The listing builds one solid part. Answer for the finished solid, in the listing's coordinates (mm). A direction names the side the tool comes from. Round coordinates to 2 decimals unless told otherwise and drop trailing zeros. Loops run counter-clockwise (first coordinate to the right, second up) from the corner with the lowest first, then second, coordinate; pieces in that order, holes last. Notation, with made-up numbers: M -31,82 L -12,82 A37 ccw -12,119 Z; hole C 82.25,-26.5 d4. An arc over 180 degrees is marked long. Put each result on its own line as item: value. Start each with the question number.
(1) Section D-D, the plane y = -30.5 is taken. Determine the outline of the cut face in (x, z), then the cut area to 3 significant figures.
(2) Flat-ended cylindrical pins translate along their axes: P1, Ø1.5, axis at y = 24, z = 3, coming from the +X side; P2, Ø1.5, axis at x = -12.5, z = 4, coming from the +Y side; P3, Ø2.5, axis at y = -23.5, z = 2.5, coming from the +X side. Find the tip coordinate at first contact, or state that the pin passes through.
(3) Section B-B, the plane y = -22 is taken. Determine the outline of the cut face in (x, z), then the cut area to 3 significant figures.
(4) Straight lines are drawn through the part: line 1 (Y direction, x = -0.5, z = 2.8) (3 decimals); line 2 (Y direction, x = 2, z = 4.75); line 3 (X direction, y = 12.5, z = 0.2) (3 decimals). For each, find the intervals that lie inside material, in ascending order.
(5) Determine the mould class of faces 3 (the face through (25, -2, 2)), 4 (the face through (0, 21.5, 3)), 5 (the face through (17.482, 29.871, 2.535)), 6 (the face through (-20.982, -28.273, 2.535)) for opening direction Y: released by +Y, released by -Y, zero draft, split by the parting line, or undercut.
(6) Section A-A, the plane z = 1.4 is taken. Count the separate pieces of the cut face and the enclosed holes in it, then the cut area to 3 significant figures.
(7) Section C-C, the plane x = -19.5 is taken. Determine the outline of the cut face in (y, z).
(8) Which of the six approach directions +Z, -Z, +X, -X, +Y, -Y give full straight-line access (tool end or side, diameter ignored) to faces 1 (the face through (-25, -2, 2)), 2 (the face through (3.5, -24, 3))?
```python
from build123d import *

# Parameters (mm, degrees)
SKETCH1_R           = 37
BOSS_EXTRUDE1_DEPTH = 5
CUT_EXTRUDE3_START  = -10
CUT_EXTRUDE3_DEPTH  = 10
FILLET2_R           = 25
FILLET3_R           = 20
SKETCH7_W           = 5
SKETCH7_H           = 5
SKETCH7_W_2         = 7
CUT_EXTRUDE4_DEPTH  = 10
SKETCH8_W           = 10
SKETCH8_H           = 7
CUT_EXTRUDE5_DEPTH  = 10


with BuildPart() as part:
    # Sketch1 → Boss-Extrude1 (new body)
    with BuildSketch(Plane.XY):
        Circle(SKETCH1_R)
    extrude(amount=BOSS_EXTRUDE1_DEPTH)

    # Sketch6 → Cut-Extrude3 (cut)
    with BuildSketch(Plane.XY.offset(5).offset(CUT_EXTRUDE3_START)):
        with BuildLine():
            Line((-25, 27.276363394), (-25, -27.276363394))
            ThreePointArc((-25, -27.276363394), (-37, 0), (-25, 27.276363394))
        make_face()
        with BuildLine():
            Line((25, -27.276363394), (25, 27.276363394))
            ThreePointArc((25, 27.276363394), (37, 0), (25, -27.276363394))
        make_face()
    extrude(amount=CUT_EXTRUDE3_DEPTH, mode=Mode.SUBTRACT)

    # Fillet2
    fillet2_edges = [part.edges().sort_by_distance(p)[0] for p in [
        (-25, 27.276363394, 2.5),
        (25, 27.276363394, 2.5),
    ]]
    fillet(fillet2_edges, radius=FILLET2_R - 0.0001)  # a hair under: the kernel refuses the full size

    # Fillet3
    fillet3_edges = [part.edges().sort_by_distance(p)[0] for p in [
        (-25, -27.276363394, 2.5),
        (25, -27.276363394, 2.5),
    ]]
    fillet(fillet3_edges, radius=FILLET3_R)

    # Sketch7 → Cut-Extrude4 (cut)
    with BuildSketch(Plane.XY.offset(5)):
        with Locations((0, 24)):
            Rectangle(SKETCH7_W, SKETCH7_H)
        with Locations((0, -23.5)):
            Rectangle(SKETCH7_W_2, SKETCH7_H)
    extrude(amount=-CUT_EXTRUDE4_DEPTH, mode=Mode.SUBTRACT)

    # Sketch8 → Cut-Extrude5 (cut)
    with BuildSketch(Plane.XY.offset(5)):
        with Locations((13, -9)):
            Rectangle(SKETCH8_W, SKETCH8_H)
    extrude(amount=-CUT_EXTRUDE5_DEPTH, mode=Mode.SUBTRACT)


solid = part.part
```
Recorded:
1. outline: M -19.03,0 L 19.03,0 L 19.03,5 L -19.03,5 Z
1. area: 190 mm²
2. P1: stops at x = 22.33
2. P2: stops at y = 34.07
2. P3: stops at x = 24.08
3. outline: M -24.16,0 L -3.5,0 L -3.5,5 L -24.16,5 Z; M 3.5,0 L 24.16,0 L 24.16,5 L 3.5,5 Z
3. area: 207 mm²
4. line 1: y = -36.997 to -26, -21 to 21.5, 26.5 to 36.995
4. line 2: y = -36.95 to -26, -21 to 21.5, 26.5 to 36.92
4. line 3: x = -24.995 to 24.995
5. face 3: zero draft
5. face 4: undercut
5. face 5: released by +Y
5. face 6: released by -Y
6. separate pieces: 1
6. enclosed holes: 3
6. area: 3,100 mm²
7. outline: M -30.02,0 L 27.64,0 L 27.64,5 L -30.02,5 Z
8. face 1: +Z, -Z, -X, +Y, -Y
8. face 2: +Z, -Z
